Input: dimensioned drawing with shaded views. Units: mm. Origin: part minimum x, y, z. A direction names the side the tool comes from. Round coordinates to 2 decimals unless told otherwise and drop trailing zeros. Order: outer loops, then holes, each group sorted by start corner. A loop starts at its lowest first (then second) coordinate and runs counter-clockwise, first axis right, second up. Notation, with made-up numbers: (66, 89.25) - (123, 89.25) arc R34 cw to (123, 120.25) - close; hole circle Ø8 at (-33, 4). An arc over 180 degrees is marked (long way). Return JSON: item names as keys, results as strings. Group by question number.
1) Ray query, line 1 (X direction, y = 39.5, z = 132.5); line 2 (Z direction, x = 254, y = 99); line 3 (Y direction, x = 237.5, z = 131). Return the intervals inside material, ascending. Write a range as from..to.
2) Contact query for flat-ended pins moving along their axis: P1, Ø1, axis at x = 243, y = 28, coming from the +Z side; P2, Ø5.5, axis at x = 269.5, y = 86, coming from the -Z side; P3, Ø9.5, axis at y = 51.5, z = 215.5, coming from the +X side. Output: stop coordinate, or through.
3) Section B-B, the plane x = 272.5. Return loops of the section in (y, z), plus the area to 3 significant figures.
4) Access query for the marked faces 5, 6, 7 and 8. Directions: +Z, -Z, +X, -X, +Y, -Y. A direction counts if a zero-diameter tool reaches every point of the face in a straight line with its end or side. Return the directions, or none.
5) Mould query, pull axis Z, two halves, no side actions, for the marked faces 1, 2, 3 and 4. Classes: pulls with the +Z half, pulls with the -Z half, needs draft (parallel to the pull), parting line crosses it, or undercut.
6) Section C-C, the plane z = 93.5. Return loops of the section in (x, y).
7) Section D-D, the plane x = 164.5. Return loops of the section in (y, z), plus the area to 3 significant figures.
8) Section A-A, the plane y = 59. Return loops of the section in (x, z), plus the area to 3 significant figures.
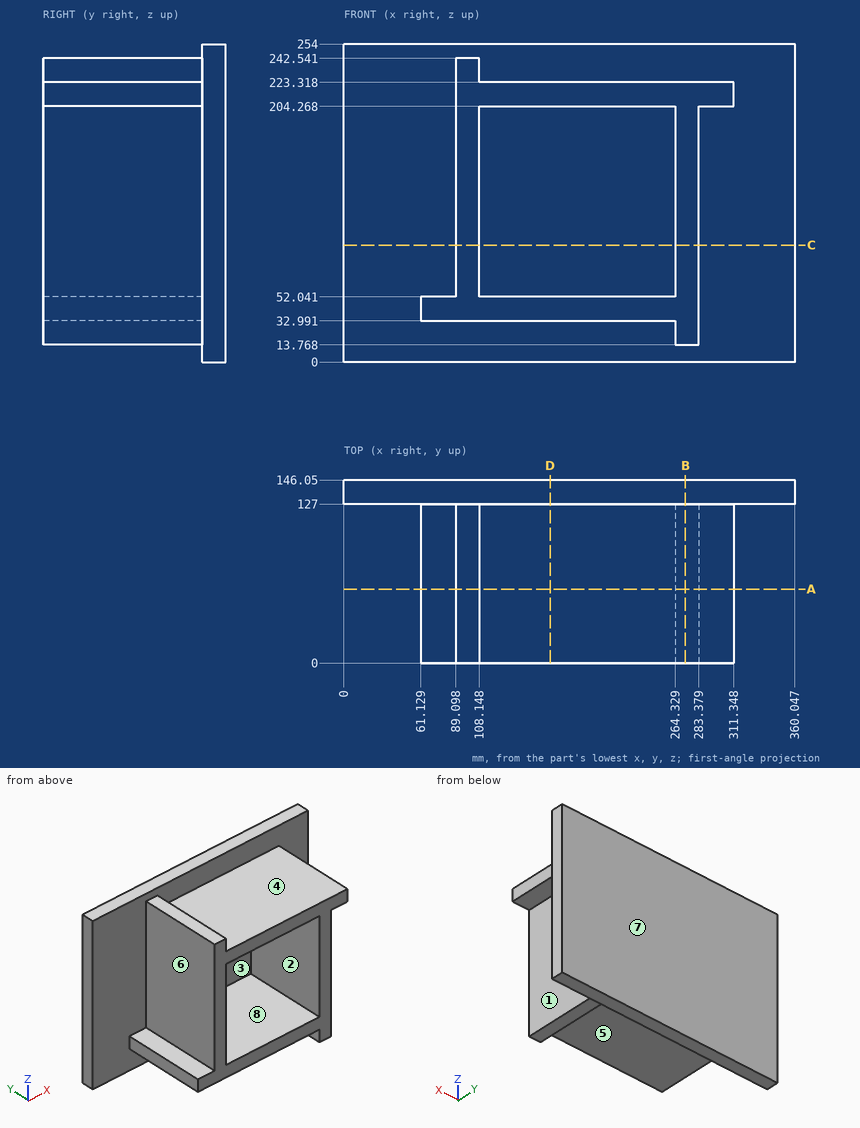
Geometry check:
{
 "1": {"line 1": "89.1..108.15, 264.33..283.38", "line 2": "32.99..52.04, 204.27..223.32", "line 3": "127..146.05"},
 "2": {"P1": "z = 223.32", "P2": "z = 13.77", "P3": "x = 311.35"},
 "3": {"outline": "(0, 13.77) - (127, 13.77) - (127, 0) - (146.05, 0) - (146.05, 254) - (127, 254) - (127, 223.32) - (0, 223.32) - close", "area": "31,500 mm2"},
 "4": {"face 5": "-Z, -X, -Y", "face 6": "+Z, -X, -Y", "face 7": "+Z, -Z, +X, -X, +Y", "face 8": "-Y"},
 "5": {"face 1": "needs draft", "face 2": "undercut", "face 3": "undercut", "face 4": "pulls with the +Z half"},
 "6": {"outline": "(0, 127) - (89.1, 127) - (89.1, 0) - (108.15, 0) - (108.15, 127) - (264.33, 127) - (264.33, 0) - (283.38, 0) - (283.38, 127) - (360.05, 127) - (360.05, 146.05) - (0, 146.05) - close"},
 "7": {"outline": "(0, 32.99) - (127, 32.99) - (127, 0) - (146.05, 0) - (146.05, 254) - (127, 254) - (127, 223.32) - (0, 223.32) - (0, 204.27) - (127, 204.27) - (127, 52.04) - (0, 52.04) - close", "area": "9,680 mm2"},
 "8": {"outline": "(61.13, 32.99) - (264.33, 32.99) - (264.33, 13.77) - (283.38, 13.77) - (283.38, 204.27) - (311.35, 204.27) - (311.35, 223.32) - (108.15, 223.32) - (108.15, 242.54) - (89.1, 242.54) - (89.1, 52.04) - (61.13, 52.04) - close; hole (108.15, 52.04) - (264.33, 52.04) - (264.33, 204.27) - (108.15, 204.27) - close", "area": "15,000 mm2"}
}
